CAD build for the part. Positions are in the model's coordinates, mm. A direction names the side the tool comes from. Give positions to 0.01 mm unless a question says otherwise; leave off trailing zeros. Write each loop counter-clockwise with the first axis right and the second up, starting at its lowest first coordinate (ties: lowest second). Pieces come first, ordered by that corner, then holes. Notation, with made-up numbers: (52.5, 40) -> (93.5, 40) arc R30 cw to (93.5, 67) -> close; hole circle Ø8 at (87.25, 0.25). An arc over 180 degrees is marked (long way). Use one line per item in the form item = value. Start each with the question number.
from build123d import *

# Parameters (mm, degrees)
F1_ANGLE = 180
F3_DEPTH = 14
F4_DEPTH = 7
F6_DEPTH = 14
F7_DEPTH = 5
F5_W     = 5
F5_H     = 10
F8_DEPTH = 6
F9_R     = 1


with BuildPart() as f1:
    # F0 (on Top) → F1 (revolve)
    with BuildSketch(Plane.XY):
        Polygon((-9.2, 14), (-9.2, 0), (-5.2, 0), (-5.2, 2.5), (-7.2, 6.5), (-7.2, 12), (0, 12), (0, 14), align=None)
    revolve(axis=Axis((0, -5.2679181099, 0), (0, -1, 0)), revolution_arc=F1_ANGLE)

    # F2 (on face) → F3 (join, through all)
    with BuildSketch(Plane(origin=(0, 14, 0), x_dir=(-1, 0, 0), z_dir=(0, 1, 0))):
        with BuildLine():
            ThreePointArc((-7.9e-09, -9.2), (-6.5053823897, -6.5053823841), (-9.2, 0))
            Line((-9.2, 0), (-9.2, -9.2))
            Line((-9.2, -9.2), (-7.9e-09, -9.2))
        make_face()
        with BuildLine():
            ThreePointArc((9.2, 0), (6.5053823841, -6.5053823897), (-7.9e-09, -9.2))
            Line((-7.9e-09, -9.2), (9.2, -9.2))
            Line((9.2, -9.2), (9.2, 0))
        make_face()
    extrude(amount=-F3_DEPTH)

    # F4 (add): a face of the model
    f4_faces = [f1.faces().sort_by_distance(p)[0] for p in [
        (-8.9687944637, 7, 0),
    ]]
    extrude(f4_faces, amount=F4_DEPTH)

    # F5 (on face) → F6 (join, through all)
    with BuildSketch(Plane(origin=(0, 14, 0), x_dir=(-1, 0, 0), z_dir=(0, 1, 0))):
        with BuildLine():
            ThreePointArc((9.2, -6.1), (12.7355339059, -4.6355339059), (14.2, -1.1))
            ThreePointArc((14.2, -1.1), (12.7355339059, 2.4355339059), (9.2, 3.9))
            Line((9.2, 3.9), (9.2, -6.1))
        make_face()
        with BuildLine():
            Line((-9.2, -6.1), (-9.2, 3.9))
            Line((-9.2, 3.9), (-11.2, 3.9))
            ThreePointArc((-11.2, 3.9), (-13.3213203436, 3.0213203436), (-14.2, 0.9))
            Line((-14.2, 0.9), (-14.2, -3.1))
            ThreePointArc((-14.2, -3.1), (-13.3213203436, -5.2213203436), (-11.2, -6.1))
            Line((-11.2, -6.1), (-9.2, -6.1))
        make_face()
    extrude(amount=-F6_DEPTH)

    # F5 (on face) → F7 (cut)
    with BuildSketch(Plane(origin=(0, 14, 0), x_dir=(-1, 0, 0), z_dir=(0, 1, 0))):
        with BuildLine():
            ThreePointArc((9.2, -6.1), (12.7355339059, -4.6355339059), (14.2, -1.1))
            ThreePointArc((14.2, -1.1), (12.7355339059, 2.4355339059), (9.2, 3.9))
            Line((9.2, 3.9), (9.2, -6.1))
        make_face()
        with BuildLine():
            Line((-9.2, -6.1), (-9.2, 3.9))
            Line((-9.2, 3.9), (-11.2, 3.9))
            ThreePointArc((-11.2, 3.9), (-13.3213203436, 3.0213203436), (-14.2, 0.9))
            Line((-14.2, 0.9), (-14.2, -3.1))
            ThreePointArc((-14.2, -3.1), (-13.3213203436, -5.2213203436), (-11.2, -6.1))
            Line((-11.2, -6.1), (-9.2, -6.1))
        make_face()
    extrude(amount=-F7_DEPTH, mode=Mode.SUBTRACT)

    # F5 (on face) → F8 (join)
    with BuildSketch(Plane(origin=(0, 14, 0), x_dir=(-1, 0, 0), z_dir=(0, 1, 0))):
        with BuildLine():
            Line((9.2, -6.1), (9.2, 3.9))
            ThreePointArc((9.2, 3.9), (4.2, -1.1), (9.2, -6.1))
        make_face()
        with BuildLine():
            ThreePointArc((9.2, -6.1), (4.2, -1.1), (9.2, 3.9))
            Line((9.2, 3.9), (9.2, 7))
            Line((9.2, 7), (-9.2, 7))
            Line((-9.2, 7), (-9.2, 3.9))
            Line((-9.2, 3.9), (-4.2, 3.9))
            Line((-4.2, 3.9), (-4.2, -6.1))
            Line((-4.2, -6.1), (-9.2, -6.1))
            Line((-9.2, -6.1), (-9.2, -9.2))
            Line((-9.2, -9.2), (9.2, -9.2))
            Line((9.2, -9.2), (9.2, -6.1))
        make_face()
        with Locations((-6.7, -1.1)):
            Rectangle(F5_W, F5_H)
    extrude(amount=F8_DEPTH)

    # F9
    f9_edges = [f1.edges().sort_by_distance(p)[0] for p in [
        (9.2, 10, 7),
        (-9.2, 10, 7),
        (9.2, 10, -9.2),
        (-9.2, 10, -9.2),
        (-7.2, 0, 7),
        (9.2, 0, 5.45),
        (9.2, 0, -7.65),
        (-9.2, 0, -7.65),
        (-9.2, 0, 5.45),
        (0, 0, -9.2),
        (0, 0, -5.2),
        (-5.2, 0, 3.5),
        (-14.2, 0, -1.1),
        (10.2, 0, -6.1),
        (13.32132, 0, -5.22132),
        (14.2, 0, -1.1),
        (13.32132, 0, 3.02132),
        (10.2, 0, 3.9),
        (7.2, 0, 7),
        (5.2, 0, 3.5),
        (0, 20, 7),
        (9.2, 20, -1.1),
        (0, 20, -9.2),
        (-9.2, 20, -1.1),
        (-14.2, 9, -1.1),
        (14.2, 9, -1.1),
        (-5.2, 2.5, 3.5),
        (-5.2, 1.25, 7),
        (5.2, 1.25, 7),
        (10.2, 9, -6.1),
        (13.32132, 9, -5.22132),
        (13.32132, 9, 3.02132),
        (10.2, 9, 3.9),
        (5.2, 2.5, 3.5),
        (0, 2.5, -5.2),
    ]]
    fillet(f9_edges, radius=F9_R)


solid = f1.part
1) Cut at D-D (y = 8.5). Give the cut face in (x, z), and give its area (3 significant figures).
2) Cut at A-A (z = 5). Give the cut face in (x, y), and give its area (3 significant figures).
3) Cut at B-B (y = 5). Give the cut face in (x, z), and give its area (3 significant figures).
4) Wall check: line 1 along X through (y, z) = (12.5, -2.5); line 2 along Y through (x, z) = (-1.25, -2.25); line 3 along X through (y, z) = (7.5, 5.5). Give the ranges that are in metal, low to high. Write a range as from..to.
5) 3-axis set-ups, long thin cutter, end or side, ignore diameter. For faces 1 (the face through (10.012, 0.285, -5.799)), 2 (the face through (8.899, 0.285, 4.816)), 3 (the face through (10.214, 8.715, 3.599)), 4 (the face through (10.186, 8.715, -5.799)): which of +Z, -Z, +X, -X, +Y, -Y reach the whole face in a straight line?
6) Pin check, flat tips, straight feed: pin 1 (1 mm diameter, centred on y = 2, z = 3.5, fed in from +X); pin 2 (2 mm diameter, centred on x = -12, z = -0.5, fed in from +Y); pin 3 (1.6 mm diameter, centred on y = 8, z = 2.5, fed in from -X). Stop position of each tip, or through.
7) Cut at C-C (y = 15). Give the cut face in (x, z).
8) Two-plate mould, pull along Y, no slides. Class faces 5 (the face through (-8.899, 9.874, 6.715)), 6 (the face through (11, 9, -1)), 7 (the face through (-7.2, 9, 3)): released by +Y, released by -Y, zero draft, split by the parting line, or undercut.
Final values:
q1.outline = (-9.2, -8.2) arc R1 ccw to (-8.2, -9.2) -> (8.2, -9.2) arc R1 ccw to (9.2, -8.2) -> (9.2, -5.97) -> (11.2, -5.97) arc R2.87 ccw to (14.07, -3.1) -> (14.07, 0.9) arc R2.87 ccw to (11.2, 3.77) -> (9.2, 3.77) -> (9.2, 6) arc R1 ccw to (8.2, 7) -> (7.2, 7) -> (7.2, 0) arc R7.2 cw to (-7.2, 0) -> (-7.2, 7) -> (-8.2, 7) arc R1 ccw to (-9.2, 6) -> (-9.2, 3.77) arc R4.87 ccw to (-9.2, -5.97) -> close
q1.area = 196 mm^2
q2.outline = (-9.2, 1) arc R1 ccw to (-8.2, 0) -> (-6.2, 0) arc R1 ccw to (-5.2, 1) -> (-5.2, 2.26) arc R1 ccw to (-5.31, 2.71) -> (-7.2, 6.5) -> (-7.2, 12) -> (7.2, 12) -> (7.2, 6.5) -> (5.31, 2.71) arc R1 ccw to (5.2, 2.26) -> (5.2, 1) arc R1 ccw to (6.2, 0) -> (8.2, 0) arc R1 ccw to (9.2, 1) -> (9.2, 19) arc R1 ccw to (8.2, 20) -> (-8.2, 20) arc R1 ccw to (-9.2, 19) -> close
q2.area = 212 mm^2
q3.outline = (-9.2, -8.2) arc R1 ccw to (-8.2, -9.2) -> (8.2, -9.2) arc R1 ccw to (9.2, -8.2) -> (9.2, -6.1) -> (11.2, -6.1) arc R3 ccw to (14.2, -3.1) -> (14.2, 0.9) arc R3 ccw to (11.2, 3.9) -> (9.2, 3.9) -> (9.2, 6) arc R1 ccw to (8.2, 7) -> (6.45, 7) -> (6.45, 0) arc R6.45 cw to (-6.45, 0) -> (-6.45, 7) -> (-8.2, 7) arc R1 ccw to (-9.2, 6) -> (-9.2, 3.9) arc R5 ccw to (-9.2, -6.1) -> close
q3.area = 227 mm^2
q4.line_1 = -9.2..9.2
q4.line_2 = 12..20
q4.line_3 = -9.2..-7.2, 7.2..9.2
q5.face_1 = -Z, +X, -Y
q5.face_2 = +Z, +X, -Y
q5.face_3 = +Z, +X, +Y
q5.face_4 = -Z, +X, +Y
q6.pin_1 = 13.34
q6.pin_2 = 9
q6.pin_3 = -13.34
q7.outline = (-9.2, -8.2) arc R1 ccw to (-8.2, -9.2) -> (8.2, -9.2) arc R1 ccw to (9.2, -8.2) -> (9.2, 6) arc R1 ccw to (8.2, 7) -> (-8.2, 7) arc R1 ccw to (-9.2, 6) -> close
q8.face_5 = zero draft
q8.face_6 = released by +Y
q8.face_7 = undercut
